Verification items for the finished model (mm, model axes). A direction names the side the tool comes from. Coordinates: 2 decimals unless noted, no trailing zeros. Order: outer loops, then holes, each group sorted by start corner. A loop starts at its lowest first (then second) coordinate and runs counter-clockwise, first axis right, second up. Notation, with made-up numbers: M 17,-38.5 L 37,-38.5 A12 ccw 37,-24.5 Z; hole C -31,9.5 d2. An arc over 180 degrees is marked long. Return JSON: item names as keys, results as strings.
```python
from build123d import *

# Parameters (mm, degrees)
SKETCH1_R           = 11
BOSS_EXTRUDE1_DEPTH = 10
SKETCH2_R           = 11
BOSS_EXTRUDE2_DEPTH = 5
SKETCH3_R           = 4
CUT_EXTRUDE1_DEPTH  = 5


with BuildPart() as part:
    # Sketch1 → Boss-Extrude1 (new body)
    with BuildSketch(Plane(origin=(-18.166693136, 0, 0), x_dir=(0, 0, -1), z_dir=(1, 0, 0))):
        with BuildLine():
            ThreePointArc((-32.070699567, 5.798220619), (-30.049213728, 4.506228855), (-27.735555242, 3.871695857))
            ThreePointArc((-27.735555242, 3.871695857), (-27.763365626, 2.885524266), (-27.735555242, 1.899352675))
            ThreePointArc((-27.735555242, 1.899352675), (-30.049213728, 1.264819676), (-32.070699567, -0.027172088))
            ThreePointArc((-32.070699567, -0.027172088), (-31.993509119, -0.556033965), (-31.90349429, -1.08286466))
            ThreePointArc((-31.90349429, -1.08286466), (-29.581699598, -1.686948368), (-27.185198138, -1.575465319))
            ThreePointArc((-27.185198138, -1.575465319), (-26.906903604, -2.521964119), (-26.575710576, -3.451275156))
            ThreePointArc((-26.575710576, -3.451275156), (-28.580049076, -4.76971169), (-30.103348944, -6.623142354))
            ThreePointArc((-30.103348944, -6.623142354), (-29.866509158, -7.102266728), (-29.61810033, -7.575496382))
            ThreePointArc((-29.61810033, -7.575496382), (-27.223270227, -7.432540112), (-24.978512054, -6.585953754))
            ThreePointArc((-24.978512054, -6.585953754), (-24.42135401, -7.400129864), (-23.819197819, -8.181612907))
            ThreePointArc((-23.819197819, -8.181612907), (-25.318017715, -10.054895223), (-26.194020408, -12.288338081))
            ThreePointArc((-26.194020408, -12.288338081), (-25.820714812, -12.67082492), (-25.438227972, -13.044130517))
            ThreePointArc((-25.438227972, -13.044130517), (-23.204785115, -12.168127824), (-21.331502799, -10.669307928))
            ThreePointArc((-21.331502799, -10.669307928), (-20.550019756, -11.271464119), (-19.735843645, -11.828622163))
            ThreePointArc((-19.735843645, -11.828622163), (-20.582430003, -14.073380336), (-20.725386273, -16.468210439))
            ThreePointArc((-20.725386273, -16.468210439), (-20.25215662, -16.716619266), (-19.773032246, -16.953459053))
            ThreePointArc((-19.773032246, -16.953459053), (-17.919601581, -15.430159185), (-16.601165047, -13.425820685))
            ThreePointArc((-16.601165047, -13.425820685), (-15.67185401, -13.757013713), (-14.725355211, -14.035308247))
            ThreePointArc((-14.725355211, -14.035308247), (-14.83683826, -16.431809706), (-14.232754552, -18.753604398))
            ThreePointArc((-14.232754552, -18.753604398), (-13.705923857, -18.843619227), (-13.177061979, -18.920809675))
            ThreePointArc((-13.177061979, -18.920809675), (-11.885070215, -16.899323836), (-11.250537217, -14.58566535))
            ThreePointArc((-11.250537217, -14.58566535), (-10.264365626, -14.613475734), (-9.278194034, -14.58566535))
            ThreePointArc((-9.278194034, -14.58566535), (-8.643661036, -16.899323836), (-7.351669272, -18.920809675))
            ThreePointArc((-7.351669272, -18.920809675), (-6.822807395, -18.843619227), (-6.2959767, -18.753604398))
            ThreePointArc((-6.2959767, -18.753604398), (-5.691892992, -16.431809706), (-5.803376041, -14.035308247))
            ThreePointArc((-5.803376041, -14.035308247), (-4.856877241, -13.757013713), (-3.927566204, -13.425820685))
            ThreePointArc((-3.927566204, -13.425820685), (-2.60912967, -15.430159185), (-0.755699006, -16.953459053))
            ThreePointArc((-0.755699006, -16.953459053), (-0.276574631, -16.716619266), (0.196655022, -16.468210439))
            ThreePointArc((0.196655022, -16.468210439), (0.053698752, -14.073380336), (-0.792887606, -11.828622163))
            ThreePointArc((-0.792887606, -11.828622163), (0.021288504, -11.271464119), (0.802771547, -10.669307928))
            ThreePointArc((0.802771547, -10.669307928), (2.676053863, -12.168127824), (4.909496721, -13.044130517))
            ThreePointArc((4.909496721, -13.044130517), (5.29198356, -12.67082492), (5.665289157, -12.288338081))
            ThreePointArc((5.665289157, -12.288338081), (4.789286464, -10.054895223), (3.290466568, -8.181612907))
            ThreePointArc((3.290466568, -8.181612907), (3.892622759, -7.400129864), (4.449780803, -6.585953754))
            ThreePointArc((4.449780803, -6.585953754), (6.694538976, -7.432540112), (9.089369079, -7.575496382))
            ThreePointArc((9.089369079, -7.575496382), (9.337777906, -7.102266728), (9.574617693, -6.623142354))
            ThreePointArc((9.574617693, -6.623142354), (8.051317825, -4.76971169), (6.046979325, -3.451275156))
            ThreePointArc((6.046979325, -3.451275156), (6.378172353, -2.521964119), (6.656466887, -1.575465319))
            ThreePointArc((6.656466887, -1.575465319), (9.052968347, -1.686948368), (11.374763038, -1.08286466))
            ThreePointArc((11.374763038, -1.08286466), (11.464777867, -0.556033965), (11.541968315, -0.027172088))
            ThreePointArc((11.541968315, -0.027172088), (9.520482476, 1.264819676), (7.20682399, 1.899352675))
            ThreePointArc((7.20682399, 1.899352675), (7.234634374, 2.885524266), (7.20682399, 3.871695857))
            ThreePointArc((7.20682399, 3.871695857), (9.520482476, 4.506228855), (11.541968315, 5.798220619))
            ThreePointArc((11.541968315, 5.798220619), (11.464777867, 6.327082497), (11.374763038, 6.853913192))
            ThreePointArc((11.374763038, 6.853913192), (9.052968347, 7.4579969), (6.656466887, 7.346513851))
            ThreePointArc((6.656466887, 7.346513851), (6.378172353, 8.29301265), (6.046979325, 9.222323687))
            ThreePointArc((6.046979325, 9.222323687), (8.051317825, 10.540760221), (9.574617693, 12.394190886))
            ThreePointArc((9.574617693, 12.394190886), (9.337777906, 12.87331526), (9.089369079, 13.346544914))
            ThreePointArc((9.089369079, 13.346544914), (6.694538976, 13.203588643), (4.449780803, 12.357002285))
            ThreePointArc((4.449780803, 12.357002285), (3.892622759, 13.171178396), (3.290466568, 13.952661439))
            ThreePointArc((3.290466568, 13.952661439), (4.789286464, 15.825943755), (5.665289157, 18.059386612))
            ThreePointArc((5.665289157, 18.059386612), (5.29198356, 18.441873452), (4.909496721, 18.815179048))
            ThreePointArc((4.909496721, 18.815179048), (2.676053863, 17.939176356), (0.802771547, 16.440356459))
            ThreePointArc((0.802771547, 16.440356459), (0.021288504, 17.04251265), (-0.792887606, 17.599670695))
            ThreePointArc((-0.792887606, 17.599670695), (0.053698752, 19.844428867), (0.196655022, 22.23925897))
            ThreePointArc((0.196655022, 22.23925897), (-0.276574631, 22.487667798), (-0.755699006, 22.724507584))
            ThreePointArc((-0.755699006, 22.724507584), (-2.60912967, 21.201207716), (-3.927566204, 19.196869216))
            ThreePointArc((-3.927566204, 19.196869216), (-4.856877241, 19.528062244), (-5.803376041, 19.806356778))
            ThreePointArc((-5.803376041, 19.806356778), (-5.691892992, 22.202858238), (-6.2959767, 24.52465293))
            ThreePointArc((-6.2959767, 24.52465293), (-6.822807395, 24.614667759), (-7.351669272, 24.691858207))
            ThreePointArc((-7.351669272, 24.691858207), (-8.643661036, 22.670372368), (-9.278194034, 20.356713882))
            ThreePointArc((-9.278194034, 20.356713882), (-10.264365626, 20.384524266), (-11.250537217, 20.356713882))
            ThreePointArc((-11.250537217, 20.356713882), (-11.885070215, 22.670372368), (-13.177061979, 24.691858207))
            ThreePointArc((-13.177061979, 24.691858207), (-13.705923857, 24.614667759), (-14.232754552, 24.52465293))
            ThreePointArc((-14.232754552, 24.52465293), (-14.83683826, 22.202858238), (-14.725355211, 19.806356778))
            ThreePointArc((-14.725355211, 19.806356778), (-15.67185401, 19.528062244), (-16.601165047, 19.196869216))
            ThreePointArc((-16.601165047, 19.196869216), (-17.919601581, 21.201207716), (-19.773032246, 22.724507584))
            ThreePointArc((-19.773032246, 22.724507584), (-20.25215662, 22.487667798), (-20.725386273, 22.23925897))
            ThreePointArc((-20.725386273, 22.23925897), (-20.582430003, 19.844428867), (-19.735843645, 17.599670695))
            ThreePointArc((-19.735843645, 17.599670695), (-20.550019756, 17.04251265), (-21.331502799, 16.440356459))
            ThreePointArc((-21.331502799, 16.440356459), (-23.204785115, 17.939176356), (-25.438227972, 18.815179048))
            ThreePointArc((-25.438227972, 18.815179048), (-25.820714812, 18.441873452), (-26.194020408, 18.059386612))
            ThreePointArc((-26.194020408, 18.059386612), (-25.318017715, 15.825943755), (-23.819197819, 13.952661439))
            ThreePointArc((-23.819197819, 13.952661439), (-24.42135401, 13.171178396), (-24.978512054, 12.357002285))
            ThreePointArc((-24.978512054, 12.357002285), (-27.223270227, 13.203588643), (-29.61810033, 13.346544914))
            ThreePointArc((-29.61810033, 13.346544914), (-29.866509158, 12.87331526), (-30.103348944, 12.394190886))
            ThreePointArc((-30.103348944, 12.394190886), (-28.580049076, 10.540760221), (-26.575710576, 9.222323687))
            ThreePointArc((-26.575710576, 9.222323687), (-26.906903604, 8.29301265), (-27.185198138, 7.346513851))
            ThreePointArc((-27.185198138, 7.346513851), (-29.581699598, 7.4579969), (-31.90349429, 6.853913192))
            ThreePointArc((-31.90349429, 6.853913192), (-31.993509119, 6.327082497), (-32.070699567, 5.798220619))
        make_face()
        with Locations(Location((-10.264365626, 2.885524266, 0), (0, 0, 180))):
            Circle(SKETCH1_R, mode=Mode.SUBTRACT)
    extrude(amount=-BOSS_EXTRUDE1_DEPTH)

    # Sketch2 → Boss-Extrude2 (add)
    with BuildSketch(Plane(origin=(-18.166693136, 0, 0), x_dir=(0, 0, -1), z_dir=(1, 0, 0))):
        with Locations((-10.264365626, 2.885524266)):
            Circle(SKETCH2_R)
    extrude(amount=-BOSS_EXTRUDE2_DEPTH)

    # Sketch3 → Cut-Extrude1 (cut)
    with BuildSketch(Plane(origin=(-18.166693136, 0, 0), x_dir=(0, 0, -1), z_dir=(1, 0, 0))):
        with Locations((-10.264365626, 2.885524266)):
            Circle(SKETCH3_R)
    extrude(amount=-CUT_EXTRUDE1_DEPTH, mode=Mode.SUBTRACT)


solid = part.part
```
Q1. Cross-section at A-A, the plane z = 19. Record the boundary of the cut face in (x, y), and give its area (3 significant figures).
Values:
{"outline": "M -28.17,-16.43 L -18.17,-16.43 L -18.17,22.2 L -28.17,22.2 L -28.17,9.57 L -23.17,9.57 L -23.17,-3.8 L -28.17,-3.8 Z", "area": "319 mm^2"}
Q2. Tool access check on faces 1 (the face through (-23.097, 6.32, -11.466)), 2 (the face through (-23.097, 15.855, 25.335)), 3 (the face through (-23.1, 13.2, 27.2)), 4 (the face through (-23.097, -15.405, 2.632)). Record the directions out of +Z, -Z, +X, -X, +Y, -Y that give a thin tool (end or side, any length) a straight path to the whole face; none if there is none.
Values:
{"face 1": "-Z, +X, -X, +Y", "face 2": "+Z, +X, -X", "face 3": "+X, -X", "face 4": "+X, -X, -Y"}
Q3. Cross-section at B-B, the plane y = -5.5. Record the boundary of the cut face in (x, z).
Values:
{"outline": "M -28.17,-8.77 L -18.17,-8.77 L -18.17,29.29 L -28.17,29.29 L -28.17,17.38 L -23.17,17.38 L -23.17,3.15 L -28.17,3.15 Z"}
Q4. Draft check along Z on faces 5 (the face through (-23.097, -4.747, 28.555)), 6 (the face through (-23.1, 12.87, -9.34)), 7 (the face through (-23.1, 19.53, 15.66)), 8 (the face through (-23.1, -1.69, -9.02)). Enter one of: pulls with the +Z half, pulls with the -Z half, needs draft (parallel to the pull), parting line crosses it, or undercut.
Values:
{"face 5": "pulls with the +Z half", "face 6": "pulls with the -Z half", "face 7": "undercut", "face 8": "undercut"}
Q5. Go/stop test with flat-tipped pins: pin 1 (24 mm diameter, centred on y = -1, z = 10, fed in from -X); pin 2 (4 mm diameter, centred on x = -19.5, y = -9, fed in from +Z); pin 3 (6.5 mm diameter, centred on y = 2.89, z = 10.26, fed in from +X); pin 4 (1.5 mm diameter, centred on x = -21.5, z = 19.5, fed in from -Y). Record where each tip stops, or that it passes through.
Values:
{"pin 1": "x = -28.17", "pin 2": "z = 29.92", "pin 3": "through", "pin 4": "y = -16.95"}
Q6. Material ranges on line 1 along Y through (x, z) = (-19.25, -3.5); line 2 along Y through (x, z) = (-23.75, 25); line 3 along Z through (x, y) = (-23, -14.5), recorded low to high.
Values:
{"line 1": "-12.58 to -8.38, -7.92 to 13.69, 14.15 to 18.35", "line 2": "-12.93 to -9.55, -6.6 to 12.37, 15.32 to 18.7", "line 3": "-0.13 to 3.33, 5.72 to 14.8, 17.2 to 20.66"}
